from build123d import *

# Parameters (mm, degrees)
F1_DEPTH = 63.5
F0_W     = 24.0836695663
F0_H     = 19.05
F2_DEPTH = 25.4
F3_DEPTH = 7.9375
F5_R     = 6.35


with BuildPart() as f1:
    # F0 (on Front) → F1 (new body, symmetric)
    with BuildSketch(Plane.XZ):
        Polygon((41.275, -9.525), (41.275, 9.525), (22.225, 9.525), (-41.275, 9.525), (-41.275, -9.525), align=None)
    extrude(amount=F1_DEPTH, both=True)

    # F0 (on Front) → F2 (join, symmetric)
    with BuildSketch(Plane.XZ):
        with Locations((72.3668347831, 52.4002)):
            Rectangle(F0_W, F0_H)
        with BuildLine():
            Line((22.225, 9.525), (41.275, 9.525))
            Line((41.275, 9.525), (41.275, 27.0002))
            ThreePointArc((41.275, 27.0002), (45.9246798487, 38.2255201513), (57.15, 42.8752))
            Line((57.15, 42.8752), (60.325, 42.8752))
            Line((60.325, 42.8752), (60.325, 61.9252))
            Line((60.325, 61.9252), (57.15, 61.9252))
            ThreePointArc((57.15, 61.9252), (43.7847811246, 59.266692673), (32.4542956671, 51.6959043329))
            ThreePointArc((32.4542956671, 51.6959043329), (24.883507327, 40.3654188754), (22.225, 27.0002))
            Line((22.225, 27.0002), (22.225, 9.525))
        make_face()
    extrude(amount=F2_DEPTH, both=True)

    # F0 (on Front) → F3 (join, symmetric)
    with BuildSketch(Plane.XZ):
        with BuildLine():
            Line((-41.275, 9.525), (22.225, 9.525))
            Line((22.225, 9.525), (22.225, 27.0002))
            ThreePointArc((22.225, 27.0002), (24.883507327, 40.3654188754), (32.4542956671, 51.6959043329))
            Line((32.4542956671, 51.6959043329), (-41.275, 9.525))
        make_face()
    extrude(amount=F3_DEPTH, both=True)

    # F0 (on Front) → F4 (revolve)
    with BuildSketch(Plane.XZ):
        Polygon((84.4086695663, 61.9252), (84.4086695663, 42.8752), (84.4086695663, 38.1), (111.125, 38.1), (111.125, 66.675), (84.4086695663, 66.675), align=None)
    revolve(axis=Axis((84.4086695663, 0, 52.3875), (0, 0, 1)))

    # F5
    f5_edges = [f1.edges().sort_by_distance(p)[0] for p in [
        (41.275, -63.5, 0),
        (-41.275, -63.5, 0),
        (-41.275, 63.5, 0),
        (41.275, 63.5, 0),
    ]]
    fillet(f5_edges, radius=F5_R)


solid = f1.part
Input: part model. Units: mm. Frame: model coordinates. A direction names the side the tool comes from. Give positions to 0.01 mm unless a question says otherwise; leave off trailing zeros. Order: outer loops, then holes, each group sorted by start corner. A loop starts at its lowest first (then second) coordinate and runs counter-clockwise, first axis right, second up. Notation, with made-up numbers: (3, -12.5) - (24, -12.5) arc R20 ccw to (24, 11.5) - close; hole circle Ø10 at (71.5, -28). An arc over 180 degrees is marked (long way). Answer as a JSON object with one key per item and string values. Group by question number.
Q1. Line query: probe 1 along X at (y, z) = (49.5, 7.5) (3 decimals); probe 2 along Z at (x, y) = (-31, -48) (3 decimals); probe 3 along Y at (x, z) = (38.5, 49). Output: solid intervals per line, ascending.
Q2. Cut plane D-D, the plane y = 17.5. Output: boundary loops of the cut face in (x, z) (3 decimals).
Q3. Cut plane C-C, the plane x = 18. Output: boundary loops of the cut face in (y, z) (1 decimal), then the cut area to 3 significant figures.
Q4. Set-up query: faces 5 (the face through (85, 0, 38.1)), 6 (the face through (22.225, 17, 18)), 7 (the face through (57.5, -2, 61.925)). Return all of +Z, -Z, +X, -X, +Y, -Y with unobstructed straight access to the full face (end or side cutting, diameter ignored); none if empty.
Q5. Mould query, pull axis X, two halves, no side actions, for faces 1 (the face through (32.73, -0.36, 51.97)), 2 (the face through (39.464, -61.59, 0.133)), 3 (the face through (1, -36, 9.525)), 4 (the face through (45.8, -0.4, 38.1)). Classes: pulls with the +X half, pulls with the -X half, needs draft (parallel to the pull), parting line crosses it, or undercut.
Q6. Cut plane B-B, the plane z = 5.5. Output: boundary loops of the cut face in (x, y) (3 decimals), then the cut area to 3 significant figures.
Q7. First-contact query: pin 1 Ø1.5 at (y, z) = (10, 52) entering from +X; pin 2 Ø15.5 at (x, z) = (45.5, 33.5) entering from -Y; pin 3 Ø15.5 at (x, z) = (56.5, 47) entering from +Y; pin 4 Ø12 at (x, z) = (50.5, 9.5) entering from +Y. Flat tips, straight axial feed; report the tip coordinate or a pass-through.
Q8. Cut plane A-A, the plane y = 0. Output: boundary loops of the cut face in (x, z) (3 decimals), then the cut area to 3 significant figures.
Results:
{
 "1": {"probe 1": "-41.275 to 41.275", "probe 2": "-9.525 to 9.525", "probe 3": "-25.4 to 25.4"},
 "2": {"outline": "(-41.275, -9.525) - (41.275, -9.525) - (41.275, 27) arc R15.875 cw to (57.15, 42.875) - (64.222, 42.875) - (64.222, 38.1) - (104.596, 38.1) - (104.596, 66.675) - (64.222, 66.675) - (64.222, 61.925) - (57.15, 61.925) arc R34.925 ccw to (22.225, 27) - (22.225, 9.525) - (-41.275, 9.525) - close"},
 "3": {"outline": "(-63.5, -9.5) - (63.5, -9.5) - (63.5, 9.5) - (7.9, 9.5) - (7.9, 43.4) - (-7.9, 43.4) - (-7.9, 9.5) - (-63.5, 9.5) - close", "area": "2,960 mm^2"},
 "4": {"face 5": "-Z, +X, +Y, -Y", "face 6": "+Z, -X, +Y", "face 7": "+Z, -X"},
 "5": {"face 1": "pulls with the -X half", "face 2": "pulls with the +X half", "face 3": "needs draft", "face 4": "undercut"},
 "6": {"outline": "(-41.275, -57.15) arc R6.35 ccw to (-34.925, -63.5) - (34.925, -63.5) arc R6.35 ccw to (41.275, -57.15) - (41.275, 57.15) arc R6.35 ccw to (34.925, 63.5) - (-34.925, 63.5) arc R6.35 ccw to (-41.275, 57.15) - close", "area": "10,400 mm^2"},
 "7": {"pin 1": "x = 109.47", "pin 2": "y = -25.4", "pin 3": "y = 25.4", "pin 4": "through"},
 "8": {"outline": "(-41.275, -9.525) - (41.275, -9.525) - (41.275, 27) arc R15.875 cw to (57.15, 42.875) - (57.692, 42.875) - (57.692, 38.1) - (111.125, 38.1) - (111.125, 66.675) - (57.692, 66.675) - (57.692, 61.925) - (57.15, 61.925) arc R34.925 ccw to (32.454, 51.696) - (-41.275, 9.525) - close", "area": "5,400 mm^2"}
}
